Input: part model. Units: mm. Frame: model coordinates. Face numbers are marked on the shaded views. A direction names the side the tool comes from. Give positions to 0.01 mm unless a question says otherwise; leave off trailing zeros. Order: outer loops, then holes, each group sorted by start corner. A loop starts at its lowest first (then second) coordinate and runs counter-clockwise, first axis right, second up. Notation, with made-up numbers: (24.5, 81.25) - (71.5, 81.25) arc R18 cw to (71.5, 87.25) - close; hole circle Ø3 at (-21, 44.25). An arc over 180 degrees is marked (long way). Answer in a Markdown table with one row per item. Add a question column.
1. Mould query, pull axis Z, two halves, no side actions, for the marked faces 1, 2 and 3. Classes: released by +Z, released by -Z, zero draft, split by the parting line, or undercut.
2. Section query A-A on y = 24. Return loops of the section in (x, z).
3. Contact query for flat-ended pins moving along their axis: pin 1 (4 mm diameter, centred on x = -15, z = -10, fed in from +Y); pin 2 (4 mm diameter, centred on y = -14.5, z = -5.5, fed in from +X); pin 3 (1.5 mm diameter, centred on x = -8, y = 6.5, fed in from -Z); pin 4 (10 mm diameter, centred on y = 13, z = -11.5, fed in from +X). Output: stop coordinate, or through.
4. Section query D-D on y = -14. Return loops of the section in (x, z).
5. Access query for the marked faces 4, 5 and 6. Directions: +Z, -Z, +X, -X, +Y, -Y. A direction counts if a zero-diameter tool reaches every point of the face in a straight line with its end or side. Return the directions, or none.
6. Section query C-C on z = -16. Return loops of the section in (x, y), and give its area (3 significant figures).
7. Ray query, line 1 (Y direction, x = -33, z = 0); line 2 (X direction, y = 24, z = -12); line 3 (X direction, y = 16, z = -6). Return the intervals inside material, ascending. Write a range as [from, to].
8. Section query B-B on x = -30.5. Return loops of the section in (y, z).
```python
from build123d import *

# Parameters (mm, degrees)
M12X1_51_D     = 10.5
M12X1_51_DEPTH = 45
M12X1_51_TIP   = 3.15451825


with BuildPart() as part:
    # Эскиз1 → Повернуть1 (revolve)
    with BuildSketch(Plane.XY, mode=Mode.PRIVATE) as revolve_1_sk:
        Polygon((0, 0), (-70, 0), (-70, -9), (-67, -12.451105222), (-67, -28), (-62, -28), (-62, -23), (-57.4, -23), (-57.4, -28), (-52.8, -28), (-52.8, -12.5), (0, -12.5), align=None)
    revolve(revolve_1_sk.sketch.rotate(Axis((-541.044005746, 0, 0), (1, 0, 0)), 270), axis=Axis((-541.044005746, 0, 0), (1, 0, 0)))

    # Сверление под метчик M12x1.51
    with Locations(Plane(origin=(0, 0, 0), x_dir=(0, 0, 1), z_dir=(1, 0, 0))):
        with Locations((0, 0)):
            Hole(M12X1_51_D / 2, depth=M12X1_51_DEPTH)
            with Locations((0, 0, -(M12X1_51_DEPTH + M12X1_51_TIP / 2))):  # 118° drill point
                Cone(0, M12X1_51_D / 2, M12X1_51_TIP, mode=Mode.SUBTRACT)


solid = part.part
```
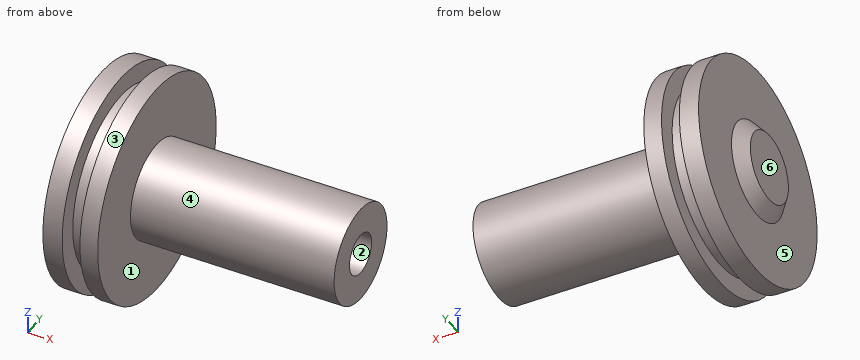
Answer:
| question | item | result |
|---|---|---|
| 1 | face 1 | zero draft |
| 1 | face 2 | undercut |
| 1 | face 3 | split by the parting line |
| 2 | outline | (-67, -14.42) - (-62, -14.42) - (-62, 14.42) - (-67, 14.42) - close; (-57.4, -14.42) - (-52.8, -14.42) - (-52.8, 14.42) - (-57.4, 14.42) - close |
| 3 | pin 1 | stops at y = 9.6 |
| 3 | pin 2 | stops at x = -52.8 |
| 3 | pin 3 | stops at z = -11.1 |
| 3 | pin 4 | stops at x = 0 |
| 4 | outline | (-67, -24.25) - (-62, -24.25) - (-62, -18.25) - (-57.4, -18.25) - (-57.4, -24.25) - (-52.8, -24.25) - (-52.8, 24.25) - (-57.4, 24.25) - (-57.4, 18.25) - (-62, 18.25) - (-62, 24.25) - (-67, 24.25) - close |
| 5 | face 4 | +X |
| 5 | face 5 | -X |
| 5 | face 6 | +Z, -Z, -X, +Y, -Y |
| 6 | outline | (-67, -22.98) - (-62, -22.98) - (-62, -16.52) - (-57.4, -16.52) - (-57.4, -22.98) - (-52.8, -22.98) - (-52.8, 22.98) - (-57.4, 22.98) - (-57.4, 16.52) - (-62, 16.52) - (-62, 22.98) - (-67, 22.98) - close |
| 6 | area | 593 mm² |
| 7 | line 1 | y = [-12.5, -5.25], [5.25, 12.5] |
| 7 | line 2 | x = [-67, -62], [-57.4, -52.8] |
| 7 | line 3 | x = [-67, -52.8] |
| 8 | outline | circle Ø25 at (0, 0); hole circle Ø10.5 at (0, 0) |
